```python
from build123d import *

# Parameters (mm, degrees)
ESQUISSE1_W                  = 52
ESQUISSE1_H                  = 40
ESQUISSE1_R                  = 14
BOSS_EXTRU_1_DEPTH           = 40
CHANFREIN1_SIZE              = 12
TROU_TARAUD_M51_AT_2_COUNT   = 2
TROU_TARAUD_M51_AT_2_PITCH   = 38
R_P_TITION_CIRCULAIRE1_COUNT = 2
R_P_TITION_CIRCULAIRE1_ANGLE = 45
R_P_TITION_CIRCULAIRE2_COUNT = 2
R_P_TITION_CIRCULAIRE2_ANGLE = 315
TROU_TARAUD_M52_D            = 4.2
TROU_TARAUD_M52_DEPTH        = 14
TROU_TARAUD_M52_TIP          = 1.2618073
CONG_1_R                     = 0.2
CHANFREIN2_SIZE              = 0.4


with BuildPart() as part:
    # Esquisse1 → Boss.-Extru.1 (new body)
    with BuildSketch(Plane.XY):
        with Locations((26, 20)):
            Rectangle(ESQUISSE1_W, ESQUISSE1_H)
        with Locations((26, 20)):
            Circle(ESQUISSE1_R, mode=Mode.SUBTRACT)
    extrude(amount=BOSS_EXTRU_1_DEPTH)

    # Chanfrein1
    chanfrein1_edges = [part.edges().sort_by_distance(p)[0] for p in [
        (0, 40, 20),
        (52, 40, 20),
    ]]
    chamfer(chanfrein1_edges, length=CHANFREIN1_SIZE)

    # Esquisse2 → Trou taraudé M51 (revolve, cut)
    with BuildSketch(Plane(origin=(7, 20, 40), x_dir=(0, -1, 0), z_dir=(1, 0, 0))):
        Polygon((0, 0), (0, 15.2618073), (2.1, 14), (2.1, 0), align=None)
    trou_taraud_m51 = revolve(axis=Axis((7, 20, 46.35), (0, 0, -1)), mode=Mode.SUBTRACT)

    # Trou taraudé M51 at 2: Trou taraudé M51 ×2
    with Locations(*[(i * TROU_TARAUD_M51_AT_2_PITCH, 0, 0) for i in range(1, TROU_TARAUD_M51_AT_2_COUNT)]):
        add(trou_taraud_m51, mode=Mode.SUBTRACT)

    # Répétition circulaire1: Trou taraudé M51 ×2 about axis
    r_p_tition_circulaire1_axis = Axis((26, 20, 0), (0, 0, 1))
    for i in range(1, R_P_TITION_CIRCULAIRE1_COUNT):
        add(trou_taraud_m51.rotate(r_p_tition_circulaire1_axis, i * R_P_TITION_CIRCULAIRE1_ANGLE / (R_P_TITION_CIRCULAIRE1_COUNT - 1)), mode=Mode.SUBTRACT)

    # Répétition circulaire1 copy 1 sketch → Répétition circulaire1 copy 1 (revolve, cut)
    with BuildSketch(Plane(origin=(39.435028843, 33.435028843, 40), x_dir=(0.707106781, -0.707106781, 0), z_dir=(0.707106781, 0.707106781, 0))):
        Polygon((0, 0), (0, 15.2618073), (2.1, 14), (2.1, 0), align=None)
    revolve(axis=Axis((39.435028843, 33.435028843, 46.35), (0, 0, -1)), mode=Mode.SUBTRACT)

    # Répétition circulaire2: Trou taraudé M51 ×2 about axis
    r_p_tition_circulaire2_axis = Axis((26, 20, 0), (0, 0, 1))
    for i in range(1, R_P_TITION_CIRCULAIRE2_COUNT):
        add(trou_taraud_m51.rotate(r_p_tition_circulaire2_axis, i * R_P_TITION_CIRCULAIRE2_ANGLE / (R_P_TITION_CIRCULAIRE2_COUNT - 1)), mode=Mode.SUBTRACT)

    # Répétition circulaire2 copy 1 sketch → Répétition circulaire2 copy 1 (revolve, cut)
    with BuildSketch(Plane(origin=(39.435028843, 6.564971157, 40), x_dir=(-0.707106781, -0.707106781, 0), z_dir=(0.707106781, -0.707106781, 0))):
        Polygon((0, 0), (0, 15.2618073), (2.1, 14), (2.1, 0), align=None)
    revolve(axis=Axis((39.435028843, 6.564971157, 46.35), (0, 0, -1)), mode=Mode.SUBTRACT)

    # Trou taraudé M52
    with Locations(Plane(origin=(0, 0, 0), x_dir=(-1, 0, 0), z_dir=(0, -1, 0))):
        with Locations((-46, -32), (-46, -8), (-6, -32), (-6, -8)):
            Hole(TROU_TARAUD_M52_D / 2, depth=TROU_TARAUD_M52_DEPTH)
            with Locations((0, 0, -(TROU_TARAUD_M52_DEPTH + TROU_TARAUD_M52_TIP / 2))):  # 118° drill point
                Cone(0, TROU_TARAUD_M52_D / 2, TROU_TARAUD_M52_TIP, mode=Mode.SUBTRACT)

    # Congé1
    cong_1_edges = [part.edges().sort_by_distance(p)[0] for p in [
        (52, 14, 40),
        (12, 20, 0),
        (0, 14, 0),
        (0, 14, 40),
        (0, 28, 20),
        (26, 40, 0),
        (46, 34, 0),
        (6, 34, 0),
        (26, 40, 40),
        (40, 40, 20),
        (12, 40, 20),
        (46, 34, 40),
        (6, 34, 40),
        (52, 28, 20),
        (52, 14, 0),
        (26, 0, 0),
        (26, 0, 40),
        (52, 0, 20),
        (0, 0, 20),
    ]]
    fillet(cong_1_edges, radius=CONG_1_R)

    # Chanfrein2
    chanfrein2_edges = [part.edges().sort_by_distance(p)[0] for p in [
        (12, 20, 40),
        (45, 22.1, 40),
        (7, 22.1, 40),
        (37.950104602, 34.919953083, 40),
        (11.080046917, 8.049895398, 40),
        (40.919953083, 8.049895398, 40),
        (14.049895398, 34.919953083, 40),
    ]]
    chamfer(chanfrein2_edges, length=CHANFREIN2_SIZE)


solid = part.part
```
Input: part model. Units: mm. Frame: model coordinates. A direction names the side the tool comes from. Round coordinates to 2 decimals unless told otherwise and drop trailing zeros. Write each loop counter-clockwise with the first axis right and the second up, starting at its lowest first coordinate (ties: lowest second). Pieces come first, ordered by that corner, then holes. Notation, with made-up numbers: (-25, 61) - (-9, 61) arc R12 ccw to (-9, 70) - close; hole circle Ø11 at (-28.5, 87.25). An arc over 180 degrees is marked (long way). Write item = value, one per line.
(1) Material intervals for probe 1 along X at (y, z) = (9.25, 8); probe 2 along X at (y, z) = (35, 35); probe 3 along Y at (x, z) = (37, 24), sorted ascending.
Geometry check:
probe_1 = 0 to 3.9, 8.1 to 17.03, 34.97 to 43.9, 48.1 to 52
probe_2 = 7 to 11.16, 13.97 to 38.03, 40.84 to 45
probe_3 = 0 to 11.34, 28.66 to 40
(2) Access query for faces 1 (the conical face through (6.27, 15.04, 31.75)), 2 (the cylindrical face through (47.05, 20.46, 32.9)). Directions: +Z, -Z, +X, -X, +Y, -Y. A direction counts if a zero-diameter tool reaches every point of the face in a straight line with its end or side. Return the directions, or none.
Geometry check:
face_1 = -Y
face_2 = +Z
(3) Section query B-B on x = 26. Output: boundary loops of the cut face in (y, z), then the cut area to 3 significant figures.
Geometry check:
outline = (0, 0.2) arc R0.2 ccw to (0.2, 0) - (5.8, 0) arc R0.2 ccw to (6, 0.2) - (6, 39.6) - (5.6, 40) - (0.2, 40) arc R0.2 ccw to (0, 39.8) - close; (34, 0.2) arc R0.2 ccw to (34.2, 0) - (39.8, 0) arc R0.2 ccw to (40, 0.2) - (40, 39.8) arc R0.2 ccw to (39.8, 40) - (34.4, 40) - (34, 39.6) - close
area = 480 mm^2
(4) Contact query for flat-ended pins moving along their axis: pin 1 Ø5.5 at (x, z) = (46, 8) entering from +Y; pin 2 Ø3.5 at (x, z) = (6, 32) entering from -Y; pin 3 Ø4 at (x, y) = (12.56, 33.44) entering from +Z. Output: stop coordinate, or through.
Geometry check:
pin_1 = 36.75
pin_2 = 14.21
pin_3 = 25.94
(5) Section query A-A on z = 14. Output: boundary loops of the cut face in (x, y), then the cut area to 3 significant figures.
Geometry check:
outline = (0, 0.2) arc R0.2 ccw to (0.2, 0) - (51.8, 0) arc R0.2 ccw to (52, 0.2) - (52, 27.92) arc R0.2 ccw to (51.94, 28.06) - (40.06, 39.94) arc R0.2 ccw to (39.92, 40) - (12.08, 40) arc R0.2 ccw to (11.94, 39.94) - (0.06, 28.06) arc R0.2 ccw to (0, 27.92) - close; hole circle Ø28 at (26, 20)
area = 1,320 mm^2
(6) Pull-direction query (Y, two-part tool) for faces 3 (the cylindrical face through (38.981, 31.385, 32.895)), 4 (the cylindrical face through (10.899, 5.286, 32.895)), 5 (the flat face through (26, 40, 20)), 6 (the cylindrical face through (46.969, 7.098, 33.863)); classes: +Y half, -Y half, draft (parallel to the pull), parting line (faces both ways), or undercut.
Geometry check:
face_3 = undercut
face_4 = undercut
face_5 = +Y half
face_6 = draft
(7) Section query C-C on z = 31. State how many separate pieces and enclosed holes the cut face has, then the cut area to 3 significant figures.
Geometry check:
separate_pieces = 1
enclosed_holes = 7
area = 1,130 mm^2
